from build123d import *

# Parameters (mm, degrees)
SKETCH_1_R          = 1.7
SKETCH_1_R_2        = 7.5
EXTRUDE_1_DEPTH     = 5
EXTRUDE_2_DEPTH     = 23
SKETCH_4_W          = 30
SKETCH_4_H          = 5
EXTRUDE_3_DEPTH     = 86.2
CHAMFER_1_SIZE      = 10
CHAMFER_2_SIZE      = 10
CHAMFER_3_SIZE      = 14
CHAMFER_5_SIZE      = 12
CHAMFER_6_SIZE      = 5
CUT_EXTRUDE_2_DEPTH = 14
CHAMFER_7_SIZE      = 6
CHAMFER_8_SIZE      = 4


with BuildPart() as part:
    # 草图1 → 凸台-拉伸1 (new body)
    with BuildSketch(Plane(origin=(0, 0, 0), x_dir=(1, 0, 0), z_dir=(0, 1, 0))):
        with BuildLine():
            Line((33.8, 21.3), (33.8, -21.3))
            Line((33.8, -21.3), (28.8, -21.3))
            Line((28.8, -21.3), (0, -21.3))
            ThreePointArc((0, -21.3), (-21.3, 0), (0, 21.3))
            Line((0, 21.3), (28.8, 21.3))
            Line((28.8, 21.3), (33.8, 21.3))
        make_face()
        with Locations(Location((0, 13.5, 0), (0, 0, 270))):
            Circle(SKETCH_1_R, mode=Mode.SUBTRACT)
        with Locations(Location((11.691342951, -6.75, 0), (0, 0, 270))):
            Circle(SKETCH_1_R, mode=Mode.SUBTRACT)
        with Locations(Location((-11.691342951, -6.75, 0), (0, 0, 270))):
            Circle(SKETCH_1_R, mode=Mode.SUBTRACT)
        with Locations(Location((0, 0, 0), (0, 0, 270))):
            Circle(SKETCH_1_R_2, mode=Mode.SUBTRACT)
    extrude(amount=EXTRUDE_1_DEPTH)

    # 草图3 → 凸台-拉伸2 (add)
    with BuildSketch(Plane(origin=(0, 5, 0), x_dir=(1, 0, 0), z_dir=(0, 1, 0))):
        with BuildLine():
            Line((33.8, 21.3), (19.384271975, 21.3))
            ThreePointArc((19.384271975, 21.3), (28.8, 0), (19.384271975, -21.3))
            Line((19.384271975, -21.3), (33.8, -21.3))
            Line((33.8, -21.3), (33.8, 21.3))
        make_face()
    extrude(amount=EXTRUDE_2_DEPTH)

    # 草图4 → 凸台-拉伸3 (add)
    with BuildSketch(Plane(origin=(33.8, 0, 0), x_dir=(0, 0, -1), z_dir=(1, 0, 0))):
        with Locations((0, 25.5)):
            Rectangle(SKETCH_4_W, SKETCH_4_H)
    extrude(amount=EXTRUDE_3_DEPTH)

    # 倒角1
    chamfer_1_edges = [part.edges().sort_by_distance(p)[0] for p in [
        (33.8, 23, 0),
    ]]
    chamfer(chamfer_1_edges, length=CHAMFER_1_SIZE)

    # 倒角2
    chamfer_2_edges = [part.edges().sort_by_distance(p)[0] for p in [
        (33.8, 0, 0),
    ]]
    chamfer(chamfer_2_edges, length=CHAMFER_2_SIZE)

    # 倒角3
    chamfer_3_edges = [part.edges().sort_by_distance(p)[0] for p in [
        (120, 25.5, -15),
        (120, 25.5, 15),
    ]]
    chamfer(chamfer_3_edges, length=CHAMFER_3_SIZE)

    # 倒角5
    chamfer_5_edges = [part.edges().sort_by_distance(p)[0] for p in [
        (28.8, 28, 0),
    ]]
    chamfer(chamfer_5_edges, length=CHAMFER_5_SIZE)

    # 倒角6
    chamfer_6_edges = [part.edges().sort_by_distance(p)[0] for p in [
        (33.8, 18.575797856, 21.3),
        (33.8, 18.575797856, -21.3),
    ]]
    chamfer(chamfer_6_edges, length=CHAMFER_6_SIZE)

    # 草图6 → 切除-拉伸2 (cut)
    with BuildSketch(Plane(origin=(0, 28, 0), x_dir=(1, 0, 0), z_dir=(0, 1, 0))):
        with BuildLine():
            Line((50.652646896, 7.091102625), (109.617699283, 7.091102625))
            Line((109.617699283, 7.091102625), (109.617699283, -7.091102625))
            Line((109.617699283, -7.091102625), (50.652646896, -7.091102625))
            ThreePointArc((50.652646896, -7.091102625), (57.743749521, 0), (50.652646896, 7.091102625))
        make_face()
    extrude(amount=-CUT_EXTRUDE_2_DEPTH, mode=Mode.SUBTRACT)

    # 倒角7
    chamfer_7_edges = [part.edges().sort_by_distance(p)[0] for p in [
        (109.617699283, 25.5, -7.091102625),
        (109.617699283, 25.5, 7.091102625),
    ]]
    chamfer(chamfer_7_edges, length=CHAMFER_7_SIZE)

    # 倒角8
    chamfer_8_edges = [part.edges().sort_by_distance(p)[0] for p in [
        (11.9, 0, 21.3),
        (-21.3, 0, 0),
        (11.9, 0, -21.3),
    ]]
    chamfer(chamfer_8_edges, length=CHAMFER_8_SIZE)


solid = part.part
Geometry: final body of the model. Coordinates: model frame, mm. A direction names the side the tool comes from. Round coordinates to 2 decimals unless told otherwise and drop trailing zeros. Write each loop counter-clockwise with the first axis right and the second up, starting at its lowest first coordinate (ties: lowest second). Pieces come first, ordered by that corner, then holes. Notation, with made-up numbers: M -19,76 L -1,76 A23 cw -1,90 Z; hole C -38,-24 d3. An arc over 180 degrees is marked long. Write item = value, one per line.
Item 1: Pin query (flat end, axial travel): P1, Ø2, axis at y = 4, z = -7, coming from the +X side; P2, Ø10, axis at x = 60, y = 23, coming from the +Z side; P3, Ø5, axis at y = 21, z = -14.5, coming from the +X side. Return the tip coordinate at first contact, or that it passes through.
Findings:
P1 = 28.8
P2 = 15
P3 = 108
Item 2: Material intervals for line 1 along Y through (x, z) = (44.5, -13.5); line 2 along Y through (x, z) = (20, 17); line 3 along X through (y, z) = (1.05, -13.5), sorted ascending. Write a range as [from, to].
Findings:
line_1 = [23, 28]
line_2 = [0, 5]
line_3 = [-12.43, -1.7], [1.7, 24.85]
Item 3: Section query C-C on z = -4. State how many separate pieces and enclosed holes the cut face has, then the cut area to 3 significant figures.
Findings:
separate_pieces = 3
enclosed_holes = 0
area = 416 mm^2
Item 4: Section query A-A on x = 101. Return loops of the section in (y, z).
Findings:
outline = M 23,-15 L 28,-15 L 28,-7.09 L 23,-7.09 Z; M 23,7.09 L 28,7.09 L 28,15 L 23,15 Z
Item 5: Access query for faces 1 (the face through (106.58, 25.54, -4.13)), 2 (the face through (61, 25, 15)), 3 (the face through (14.1, 2, 19.3)). Directions: +Z, -Z, +X, -X, +Y, -Y. A direction counts if a zero-diameter tool reaches every point of the face in a straight line with its end or side. Return the directions, or none.
Findings:
face_1 = +Y, -Y
face_2 = +Z, +X, +Y, -Y
face_3 = +Z, +X, -X, -Y
Item 6: Pull-direction query (X, two-part tool) for faces 4 (the face through (-17.49, 0.194, 0.385)), 5 (the face through (0.51, 2.46, -11.88)), 6 (the face through (8, 0, 0)), 7 (the face through (78, 26, 7.091)); classes: pulls with the +X half, pulls with the -X half, needs draft (parallel to the pull), parting line crosses it, or undercut.
Findings:
face_4 = pulls with the -X half
face_5 = undercut
face_6 = needs draft
face_7 = undercut
Item 7: Section query B-B on x = 52. Return loops of the section in (y, z), then the cut area to 3 significant figures.
Findings:
outline = M 23,-15 L 28,-15 L 28,-7.09 L 23,-7.09 Z; M 23,-6.96 L 28,-6.96 L 28,6.96 L 23,6.96 Z; M 23,7.09 L 28,7.09 L 28,15 L 23,15 Z
area = 149 mm^2
